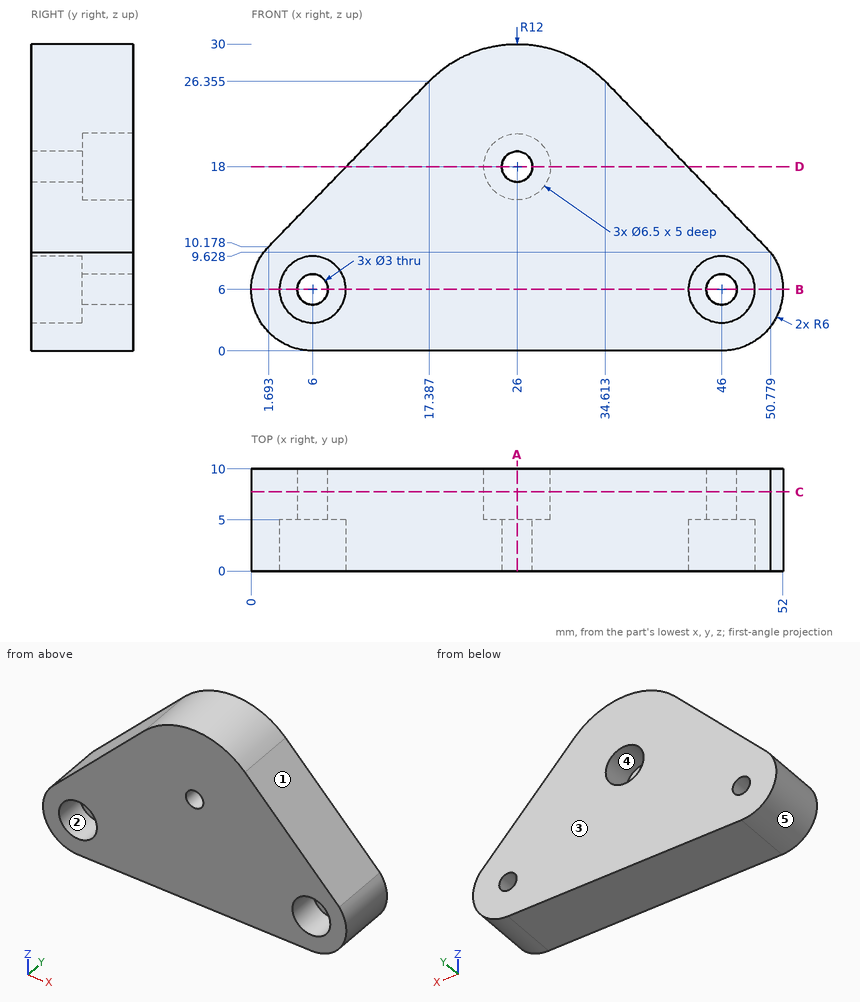
The drawing under review shows one solid part. Ordinate dimensions are in mm from its lowest x, y, z. A direction names the side the tool comes from. Round coordinates to 2 decimals unless told otherwise and drop trailing zeros. Loops run counter-clockwise (first coordinate to the right, second up) from the corner with the lowest first, then second, coordinate; pieces in that order, holes last.
Item 1: Clearance check with flat-ended pins moving along their axes: pin 1 Ø6 at (y, z) = (4, 3) entering from -X; pin 2 Ø3.5 at (x, z) = (46, 6) entering from -Y. State where each tip first meets the part, or that it passes through.
Determined:
pin 1: stops at x = 0
pin 2: stops at y = 5
Item 2: Take a section at A-A (x = 26). Write out the cut boundary in (y, z).
Determined:
outline: (0, 0) - (10, 0) - (10, 14.75) - (5, 14.75) - (5, 16.5) - (0, 16.5) - close; (0, 19.5) - (5, 19.5) - (5, 21.25) - (10, 21.25) - (10, 30) - (0, 30) - close
Item 3: For the marked faces 1 and 2, list the 3-axis set-ups (+Z, -Z, +X, -X, +Y, -Y) from which the entire face can be reached by the end or side of a thin tool; tool diameter is ignored.
Determined:
face 1: +Z, +X, +Y, -Y
face 2: -Y
Item 4: For line 1 (X direction, y = 7.8, z = 6); line 2 (X direction, y = 3.4, z = 6); line 3 (X direction, y = 6.5, z = 18), list the stretches that pass through material, from the lowest coordinate up.
Determined:
line 1: x = 0 to 4.5, 7.5 to 44.5, 47.5 to 52
line 2: x = 0 to 2.75, 9.25 to 42.75, 49.25 to 52
line 3: x = 9.28 to 22.75, 29.25 to 42.69
Item 5: Take a section at B-B (z = 6). Write out the cut boundary in (x, y).
Determined:
outline: (0, 0) - (2.75, 0) - (2.75, 5) - (4.5, 5) - (4.5, 10) - (0, 10) - close; (7.5, 5) - (9.25, 5) - (9.25, 0) - (42.75, 0) - (42.75, 5) - (44.5, 5) - (44.5, 10) - (7.5, 10) - close; (47.5, 5) - (49.25, 5) - (49.25, 0) - (52, 0) - (52, 10) - (47.5, 10) - close
Item 6: Mouldability with a two-part tool opening along X and no side actions: class the marked faces 3, 4 and 5 as released by +X, released by -X, zero draft, split by the parting line, or undercut.
Determined:
face 3: zero draft
face 4: undercut
face 5: released by -X
Item 7: Take a section at D-D (z = 18). Write out the cut boundary in (x, y).
Determined:
outline: (9.28, 0) - (24.5, 0) - (24.5, 5) - (22.75, 5) - (22.75, 10) - (9.28, 10) - close; (27.5, 0) - (42.69, 0) - (42.69, 10) - (29.25, 10) - (29.25, 5) - (27.5, 5) - close
Item 8: Take a section at C-C (y = 7.75). Give the number of separate pieces and of enclosed holes in the cut face, then the cut area to 3 significant figures.
Determined:
separate pieces: 1
enclosed holes: 3
area: 1,040 mm2
